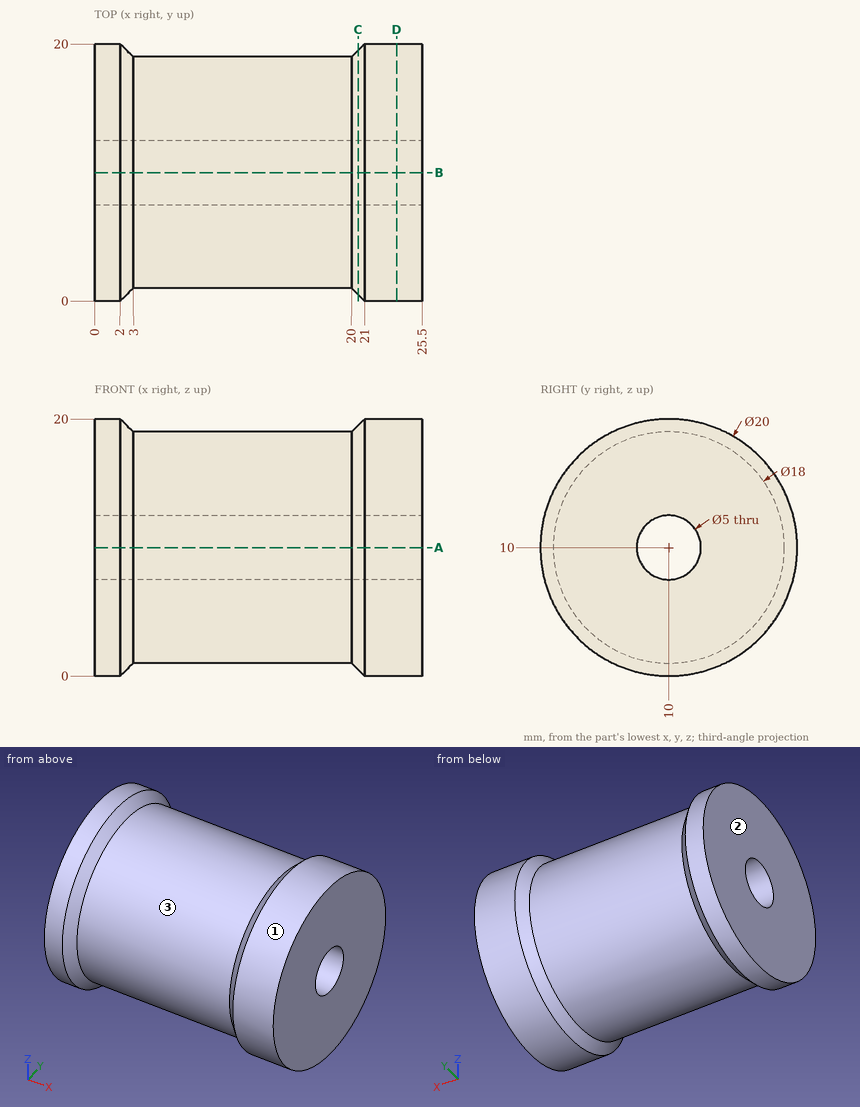
The drawing under review shows one solid part. Ordinate dimensions are in mm from its lowest x, y, z. Coordinates: 2 decimals unless noted, no trailing zeros. Order: outer loops, then holes, each group sorted by start corner. A loop starts at its lowest first (then second) coordinate and runs counter-clockwise, first axis right, second up. Notation, with made-up numbers: M 35.25,-1 L 61.25,-1 A22 ccw 61.25,21 Z; hole C 41,84.25 d4. An arc over 180 degrees is marked long. Use a Markdown table: item, result.
(1) Add section A-A (z = 10). Give the boundary of the cut face in (x, y), then the cut area to 4 significant figures.
Worked answers:
| item | result |
|---|---|
| outline | M 0,0 L 2,0 L 3,1 L 20,1 L 21,0 L 25.5,0 L 25.5,7.5 L 0,7.5 Z; M 0,12.5 L 25.5,12.5 L 25.5,20 L 21,20 L 20,19 L 3,19 L 2,20 L 0,20 Z |
| area | 346.5 mm2 |
(2) Add section C-C (x = 20.5). Give the boundary of the cut face in (y, z).
Worked answers:
| item | result |
|---|---|
| outline | C 10,10 d19; hole C 10,10 d5 |
(3) Add section D-D (x = 23.5). Give the boundary of the cut face in (y, z).
Worked answers:
| item | result |
|---|---|
| outline | C 10,10 d20; hole C 10,10 d5 |
(4) For P1, Ø8, axis at x = 11.5, z = 8, coming from the +Y side; P2, Ø6, axis at y = 10, z = 10, coming from the +X side; P3, Ø12, axis at x = 12.5, z = 8, coming from the -Y side; P4, Ø1, axis at x = 15.5, z = 12.5, coming from the -Y side, all flat-tipped, find the tip position at first contact; note any pin that passes through.
Worked answers:
| item | result |
|---|---|
| P1 | stops at y = 19 |
| P2 | stops at x = 25.5 |
| P3 | stops at y = 1 |
| P4 | stops at y = 1.23 |
(5) Wall thickness on probe 1 along Y at (x, z) = (13.25, 12.25); probe 2 along Z at (x, y) = (6.5, 8.25); probe 3 along Y at (x, z) = (20.25, 10): over which ranges is each line inside the solid? List them lowest first.
Worked answers:
| item | result |
|---|---|
| probe 1 | y = 1.29 to 8.91, 11.09 to 18.71 |
| probe 2 | z = 1.17 to 8.21, 11.79 to 18.83 |
| probe 3 | y = 0.75 to 7.5, 12.5 to 19.25 |
(6) Draft analysis for pull direction X (two halves, no side actions). For the marked faces 1, 2 and 3, state which applies: released by +X, released by -X, zero draft, split by the parting line, or undercut.
Worked answers:
| item | result |
|---|---|
| face 1 | zero draft |
| face 2 | released by -X |
| face 3 | undercut |
